from build123d import *

# Parameters (mm, degrees)
F0_R            = 115.75
F0_R_2          = 96
F1_DEPTH        = 15
F3_D            = 8.5
F3_COPIES_COUNT = 10


# Not quite as in the source:
# - a pattern or mirror of a feature is missing from the dataset's text; its kind, count and spacing are read off the source's solid


with BuildPart() as f1:
    # F0 (on Top) → F1 (new body)
    with BuildSketch(Plane.XY):
        Circle(F0_R)
        Circle(F0_R_2, mode=Mode.SUBTRACT)
    extrude(amount=F1_DEPTH)

    # F3 (through all)
    with Locations(Plane.XY.offset(15)):
        with Locations((0, 105)):
            f3 = Hole(F3_D / 2)

    # F3_copies: F3 ×10 about axis
    f3_copies_axis = Axis((0, 0, 0), (0, 0, 1))
    for i in range(1, F3_COPIES_COUNT):
        add(f3.rotate(f3_copies_axis, i * 360 / F3_COPIES_COUNT), mode=Mode.SUBTRACT)


solid = f1.part
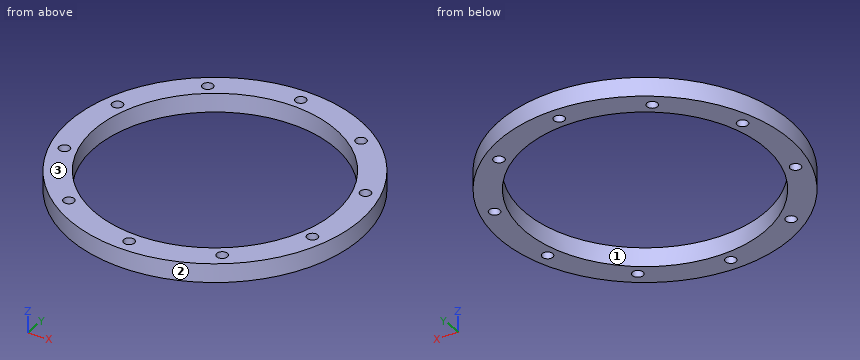
Geometry: final body of the model. Coordinates: model frame, mm. Face numbers are marked on the shaded views. Give positions to 0.01 mm unless a question says otherwise; leave off trailing zeros. Write each loop counter-clockwise with the first axis right and the second up, starting at its lowest first coordinate (ties: lowest second). Pieces come first, ordered by that corner, then holes.
(1) Mould query, pull axis X, two halves, no side actions, for the marked faces 1, 2 and 3. Classes: released by +X, released by -X, zero draft, split by the parting line, or undercut.
(2) Ray query, line 1 (Y direction, x = 0, z = 7.25); line 2 (X direction, y = -34, z = 13.75); line 3 (Y direction, x = -96.5, z = 10). Return the intervals inside material, ascending.
(3) Cut plane A-A, the plane x = 0. Return loops of the section in (y, z), then the cut area to 4 significant figures.
(4) Cut plane C-C, the plane x = 90.5. Return loops of the section in (y, z).
(5) Cut plane B-B, the plane y = 0. Return loops of the section in (x, z).
(6) Cut plane D-D, the plane z = 6. Give the number of separate pieces and of enclosed holes in the cut face, then the cut area to 3 significant figures.
(7) First-contact query: P1, Ø5, axis at x = 27, z = 8, coming from the -Y side; P2, Ø5, axis at x = 99.86, y = -32.45, coming from the +Z side; P3, Ø6, axis at y = 18, z = 7.5, coming from the -X side; P4, Ø4, axis at y = 26.5, z = 1.5, coming from the -X side. Flat tips, straight axial feed; report the tip coordinate or a pass-through.
Values follow:
1. face 1: undercut
1. face 2: split by the parting line
1. face 3: zero draft
2. line 1: y = -115.75 to -109.25, -100.75 to -96, 96 to 100.75, 109.25 to 115.75
2. line 2: x = -110.64 to -103.82, -95.9 to -89.78, 89.78 to 95.9, 103.82 to 110.64
2. line 3: y = -63.92 to -35.05, -29.85 to 29.85, 35.05 to 63.92
3. outline: (-115.75, 0) - (-109.25, 0) - (-109.25, 15) - (-115.75, 15) - close; (-100.75, 0) - (-96, 0) - (-96, 15) - (-100.75, 15) - close; (96, 0) - (100.75, 0) - (100.75, 15) - (96, 15) - close; (109.25, 0) - (115.75, 0) - (115.75, 15) - (109.25, 15) - close
3. area: 337.5 mm2
4. outline: (-72.17, 0) - (-32.03, 0) - (-32.03, 15) - (-72.17, 15) - close; (32.03, 0) - (72.17, 0) - (72.17, 15) - (32.03, 15) - close
5. outline: (-115.75, 0) - (-96, 0) - (-96, 15) - (-115.75, 15) - close; (96, 0) - (115.75, 0) - (115.75, 15) - (96, 15) - close
6. separate pieces: 1
6. enclosed holes: 11
6. area: 12,600 mm2
7. P1: stops at y = -113.13
7. P2: passes through
7. P3: stops at x = -114.77
7. P4: stops at x = -113.13
